Geometry check sheet. Reference: the model listing, model coordinates, mm. Face numbers are marked on the shaded views. Give positions to 0.01 mm unless a question says otherwise; leave off trailing zeros. Loops run counter-clockwise (first coordinate to the right, second up) from the corner with the lowest first, then second, coordinate; pieces in that order, holes last. Notation, with made-up numbers: (-16, -31) -> (8, -31) arc R7 cw to (8, -25) -> close; hole circle Ø5 at (64, 2). An arc over 180 degrees is marked (long way). One line per question, with ' | ' between items.
Autodesk Inventor part; units mm, degrees
ref_plane "YZ Plane" through (0, 0, 0) normal (1, 0, 0) x (0, 1, 0)
ref_plane "XZ Plane" through (0, 0, 0) normal (0, 1, 0) x (-1, 0, 0)
ref_plane "XY Plane" through (0, 0, 0) normal (0, 0, 1) x (1, 0, 0)
sketch "Sketch1" plane through (0, 0, 0) normal (0, 0, 1) x (1, 0, 0)
  line L0 (-2, 0) -> (35, 0)
  line L1 (35, 0) -> (35, 4)
  line L2 (35, 4) -> (3.125, 4)
  line L3 (3.125, 4) -> (2.3581, 4)
  line L4 (2.3581, 4) -> (0, 4)
  line L5 (0, 4) -> (0, 6.5)
  line L6 (0, 6.5) -> (-8, 6.5)
  line L7 (-8, 6.5) -> (-8, 3.4641)
  line L8 (-8, 3.4641) -> (-4, 3.4641)
  line L9 (-4, 3.4641) -> (-2, 0)
  line L10 (-12.3, 0) -> (47.9, 0)
  line L11 (0, -0.65) -> (0, 8.45)
  line L12 (3.125, 4) -> (0, 4) construction
  dimension "d1" = 31.875
  dimension "d2" = 0.7669
  dimension "d3" = 8
  dimension "d4" = 4
  dimension "d5" = 60
  dimension "d6" = 8
  dimension "d7" = 8
  dimension "d8" = 6.9282
  dimension "d9" = 13
  dimension "d26" = 35
revolve "Body" add sketch "Sketch1" angle 360 about axis through (-2, 0, 0) along (1, 0, 0)
sketch "Sketch2" plane through (-8, 0, 0) normal (-1, 0, 0) x (0, 0, 1)
  circle A0 centre (0, 0) radius 3.4641
  line L0 (0, -7.8) -> (0, 10.4)
  line L1 (-7.8, 0) -> (10.4, 0)
  line L2 (3.4641, 0) -> (1.7321, -3)
  line L3 (1.7321, -3) -> (-1.7321, -3)
  line L4 (-1.7321, -3) -> (-3.4641, 0)
  line L5 (-3.4641, 0) -> (-1.7321, 3)
  line L6 (-1.7321, 3) -> (1.7321, 3)
  line L7 (1.7321, 3) -> (3.4641, 0)
extrude "Slot" add sketch "Sketch2" against normal up to next contours L7 A0 | A0 L2 | L6 L0 A0 | A0 L0 L3 | L0 L6 A0 | A0 L3 L0 | L4 A0 | A0 L5
fillet "Fillet1" radius 0.8 1 edges at (-8, -6.5, 0)
thread "Thread"
chamfer "Chamfer1" distance 0.7668 distance2 0.7668 1 edges at (35, -4, 0) measured on face at (35, -0.4013, -0.6579)
equation "\"d1\" = GEL"
equation "\"d3\" = KOH"
equation "\"d4\" = INTI"
equation "\"d6\" = GD"
equation "\"d7\" = BDM"
equation "\"d8\" = 1.1547 * SW"
equation "\"d9\" = KOD"
equation "\"d26\" = NLG"
equation "\"d17\" = RR"
equation "\"d13\" = GEL"
equation "\"d15\" = -0.5 * SPD + 0.5 * GD"
equation "\"d16\" = GUL"
equation "\"GD\" = NND"
equation "\"NLG\" = 35"
equation "\"GEL\" = 31.875"
equation "\"KOD\" = 13"
equation "\"KOH\" = NND"
equation "\"INTI\" = 4"
equation "\"GAL\" = 0.61345 * TPU"
equation "\"GUL\" = 0.61345 * TPU"
equation "\"BDM\" = NND"
equation "\"SW\" = 6"
equation "\"RR\" = 0.1 * NND"
equation "\"SPD\" = NND - 1.2269 * TPU"
equation "\"TOA\" = 30deg"
equation "\"PTC\" = TPU"
equation "\"GD1\" = THREADDIA - 1.2269 * TPU"
equation "\"TPU\" = 1.25"
equation "\"THREADDIA\" = 8"
equation "\"FAWI\" = 45deg"
equation "\"E0\" = 1.155 * SW"
equation "\"NND\" = 8"
properties part number "BS 4168 - M8 x 35"
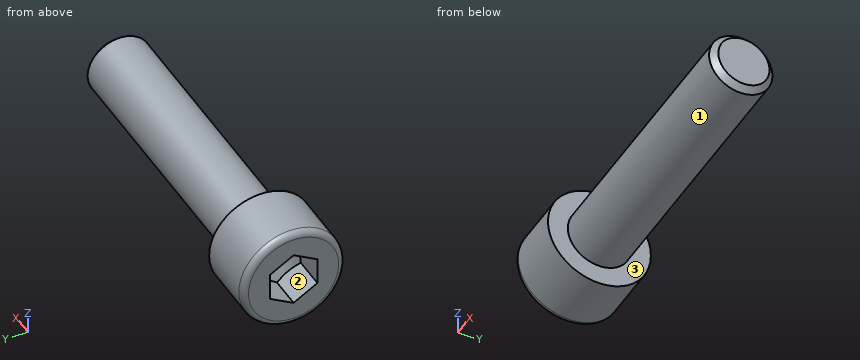
Item 1: Scan lines: probe 1 along Y at (x, z) = (3, -0.25); probe 2 along X at (y, z) = (-4.5, -1.25); probe 3 along Y at (x, z) = (8, 2.75). Record each from-to range of solid material in increasing order.
Result:
probe 1: -3.99 to 3.99 | probe 2: -8 to 0 | probe 3: -2.9 to 2.9
Item 2: Release check for a two-part mould opening along Y. For the marked faces 1, 2 and 3 record: pulls with the +Y half, pulls with the -Y half, needs draft (parallel to the pull), parting line crosses it, or undercut.
Result:
face 1: parting line crosses it | face 2: undercut | face 3: needs draft
Item 3: Depth check by flat-ended pin: pin 1 Ø6 at (x, y) = (4, 0) entering from -Z; pin 2 Ø1 at (x, z) = (-5, 1) entering from -Y; pin 3 Ø2 at (x, y) = (10.5, -3) entering from +Z. Enter the tip coordinate at first touch or a pass-through.
Result:
pin 1: z = -4 | pin 2: y = -6.48 | pin 3: z = 3.46
Item 4: Sectioned sample at A-A (x = 31.5). Record the cut outline in (y, z).
Result:
outline: circle Ø8 at (0, 0)
